Here's how the part is built. I have some questions about the finished solid (model axes, mm). Face numbers are marked on the shaded views. A direction names the side the tool comes from. Coordinates: 2 decimals unless noted, no trailing zeros. Write each loop counter-clockwise with the first axis right and the second up, starting at its lowest first coordinate (ties: lowest second). Pieces come first, ordered by that corner, then holes. Notation, with made-up numbers: M 34.25,17.5 L 40.25,17.5 A10 ccw 40.25,26.5 Z; hole C 82,61.5 d11. An arc over 180 degrees is marked long. Use one line per item in the form item = value. Start each with the question number.
1. I'm going to push flat-ended pins straight in: pin 1 Ø6.5 at (x, y) = (-28.36, -20.74) entering from -Z; pin 2 Ø1 at (x, y) = (12.5, 9) entering from +Z; pin 3 Ø1 at (x, z) = (16.5, 75) entering from +Y. Where does each tip first touch, or does it pass through?
2. Please list where these lines run through material, in increasing order: line 1 along Z through (x, y) = (13, -11); line 2 along Z through (x, y) = (-18.5, 14); line 3 along X through (y, z) = (24, 37). Write a range as [from, to].
3. I want a section at B-B, the plane x = -11.5. List the corners of the cut face in (y, z) for me.
4. On a 3-axis mill with a long thin cutter (end or side, diameter ignored), from which of +Z, -Z, +X, -X, +Y, -Y can I reach the whole of each face in a straight line? I mean the marked faces 1 and 2. Say none if no direction works.
5. I want a section at D-D, the plane z = 139. List the corners of the cut face in (x, y) for me, plus the area to 3 significant figures.
6. I want a section at C-C, the plane y = 11. List the corners of the cut face in (x, z) for me, plus the area to 3 significant figures.
from build123d import *

# Parameters (mm, degrees)
SKETCH1_W            = 57
SKETCH1_H            = 57
BOSS_EXTRUDE1_DEPTH  = 123
SKETCH2_W            = 10
SKETCH2_H            = 10
CUT_EXTRUDE1_DEPTH   = 118
LPATTERN1_COUNT      = 2
LPATTERN1_PITCH      = 47
LPATTERN1_COUNT_DIR2 = 2
LPATTERN1_PITCH_DIR2 = 47
SKETCH3_R            = 2.5
CUT_EXTRUDE2_DEPTH   = 50
LPATTERN2_COUNT      = 2
LPATTERN2_PITCH      = 47
LPATTERN2_COUNT_DIR2 = 2
LPATTERN2_PITCH_DIR2 = 47
FILLET1_R            = 5
SKETCH5_R            = 19.05
BOSS_EXTRUDE3_DEPTH  = 1.5
SKETCH4_R            = 4
BOSS_EXTRUDE2_DEPTH  = 28.5


with BuildPart() as part:
    # Sketch1 → Boss-Extrude1 (new body)
    with BuildSketch(Plane.XY):
        with Locations((-4.861204013, 2.764214047)):
            Rectangle(SKETCH1_W, SKETCH1_H)
    extrude(amount=BOSS_EXTRUDE1_DEPTH)

    # Sketch2 → Cut-Extrude1 (cut)
    with BuildSketch(Plane(origin=(0, 0, 0), x_dir=(-1, 0, 0), z_dir=(0, 0, -1))):
        with Locations((-18.638795987, 26.264214047)):
            Rectangle(SKETCH2_W, SKETCH2_H)
    cut_extrude1 = extrude(amount=-CUT_EXTRUDE1_DEPTH, mode=Mode.SUBTRACT)

    # LPattern1: Cut-Extrude1 2 × 2
    with Locations(*[(-i * LPATTERN1_PITCH, -j * LPATTERN1_PITCH_DIR2, 0) for i in range(LPATTERN1_COUNT) for j in range(LPATTERN1_COUNT_DIR2) if (i, j) != (0, 0)]):
        add(cut_extrude1, mode=Mode.SUBTRACT)

    # Sketch3 → Cut-Extrude2 (cut)
    with BuildSketch(Plane.XY.offset(123)):
        with Locations((-28.361204013, 26.264214047)):
            Circle(SKETCH3_R)
    cut_extrude2 = extrude(amount=-CUT_EXTRUDE2_DEPTH, mode=Mode.SUBTRACT)

    # LPattern2: Cut-Extrude2 2 × 2
    with Locations(*[(i * LPATTERN2_PITCH, -j * LPATTERN2_PITCH_DIR2, 0) for i in range(LPATTERN2_COUNT) for j in range(LPATTERN2_COUNT_DIR2) if (i, j) != (0, 0)]):
        add(cut_extrude2, mode=Mode.SUBTRACT)

    # Fillet1
    fillet1_edges = [part.edges().sort_by_distance(p)[0] for p in [
        (-33.361204013, 21.264214047, 59),
        (-23.361204013, 21.264214047, 59),
        (-23.361204013, 31.264214047, 59),
        (13.638795987, 31.264214047, 59),
        (13.638795987, 21.264214047, 59),
        (23.638795987, 21.264214047, 59),
        (23.638795987, -25.735785953, 120.5),
        (23.638795987, -15.735785953, 59),
        (13.638795987, -15.735785953, 59),
        (13.638795987, -25.735785953, 59),
        (-23.361204013, -25.735785953, 59),
        (-23.361204013, -15.735785953, 59),
        (-33.361204013, -15.735785953, 59),
        (-33.361204013, -25.735785953, 120.5),
        (-33.361204013, 31.264214047, 120.5),
        (23.638795987, 31.264214047, 120.5),
    ]]
    fillet(fillet1_edges, radius=FILLET1_R - 0.0001)  # a hair under: the kernel refuses the full size

    # Sketch5 → Boss-Extrude3 (add)
    with BuildSketch(Plane.XY.offset(123)):
        with Locations((-4.861204013, 2.764214047)):
            Circle(SKETCH5_R)
    extrude(amount=BOSS_EXTRUDE3_DEPTH)

    # Sketch4 → Boss-Extrude2 (add)
    with BuildSketch(Plane.XY.offset(123)):
        with Locations(Location((-4.861204013, 2.764214047, 0), (0, 0, 180))):
            Circle(SKETCH4_R)
    extrude(amount=BOSS_EXTRUDE2_DEPTH)


solid = part.part
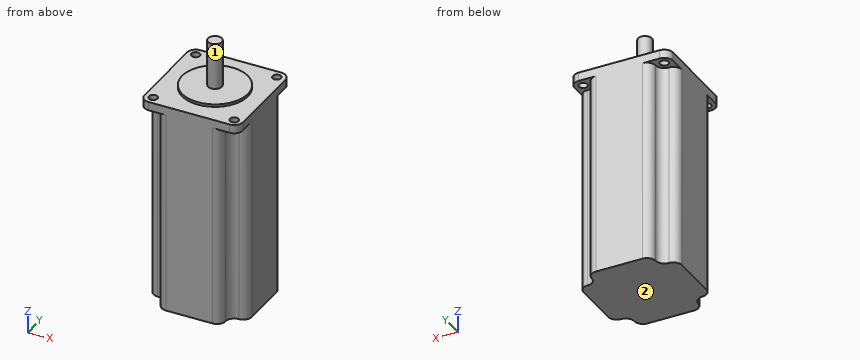
Answer list:
q1.pin_1 = 118
q1.pin_2 = 124.5
q1.pin_3 = 22.02
q2.line_1 = [0, 123]
q2.line_2 = [0, 124.5]
q2.line_3 = [-23.9, 14.18]
q3.outline = M -25.74,0 L 31.26,0 L 31.26,123 L 20.62,123 L 20.62,124.5 L -15.09,124.5 L -15.09,123 L -25.74,123 Z
q4.face_1 = +Z
q4.face_2 = -Z, +X, -X, +Y, -Y
q5.outline = C -4.86,2.76 d8
q5.area = 50.3 mm²
q6.outline = M -33.36,0 L 23.64,0 L 23.64,123 L 12.32,123 L 12.32,124.5 L -22.04,124.5 L -22.04,123 L -33.36,123 Z
q6.area = 7,060 mm²
